Part model, mm, in its own coordinate system. Face numbers are marked on the shaded views. A direction names the side the tool comes from. Coordinates: 2 decimals unless noted, no trailing zeros. Order: outer loops, then holes, each group sorted by start corner. A loop starts at its lowest first (then second) coordinate and runs counter-clockwise, first axis right, second up.
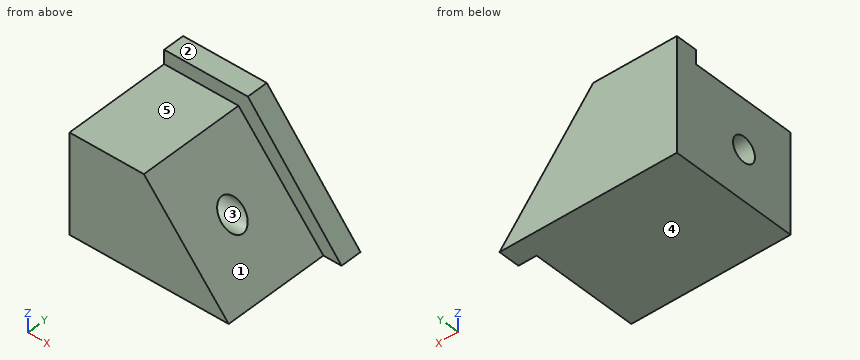
from build123d import *

# Parameters (mm, degrees)
F1_DEPTH = 76.2
F2_DEPTH = 12.7
F3_R     = 7.356687
F4_DEPTH = 104.797916


with BuildPart() as f1:
    # F0 (on Front) → F1 (new body)
    with BuildSketch(Plane.XZ):
        Polygon((0, 58.801956), (0, 0), (94.055586, 0), (43.929327, 58.801956), align=None)
    extrude(amount=F1_DEPTH)

    # F0 (on Front) → F2 (join)
    with BuildSketch(Plane.XZ):
        Polygon((0, 67.064524), (0, 58.801956), (43.929327, 58.801956), (94.055586, 0), (104.796916, 0), (49.437713, 67.064524), align=None)
    extrude(amount=F2_DEPTH)

    # F3 (on Right) → F4 (cut, through all)
    with BuildSketch(Plane.YZ):
        with Locations((-44.999432, 29.680481)):
            Circle(F3_R)
    extrude(amount=F4_DEPTH, mode=Mode.SUBTRACT)


solid = f1.part
Q1. Cut at C-C on x = 15.5. Write the cut outline in (y, z), and give its area (3 significant figures).
Results list:
outline: (-76.2, 0) - (0, 0) - (0, 67.06) - (-12.7, 67.06) - (-12.7, 58.8) - (-76.2, 58.8) - close; hole circle Ø14.71 at (-45, 29.68)
area: 4,420 mm2
Q2. Cut at D-D on z = 52. Write the cut outline in (x, y).
Results list:
outline: (0, -76.2) - (49.73, -76.2) - (49.73, -12.7) - (61.87, -12.7) - (61.87, 0) - (0, 0) - close
Q3. Pin check, flat tips, straight feed: pin 1 Ø1 at (x, y) = (87.5, -61.5) entering from +Z; pin 2 Ø8 at (y, z) = (-42.5, 47.5) entering from +X. Stop position of each tip, or through.
Results list:
pin 1: stops at z = 8.28
pin 2: stops at x = 56.97
Q4. Mould opens along Z. For the marked faces 3, 4 and 5 say: pulls with the +Z half, pulls with the -Z half, needs draft (parallel to the pull), parting line crosses it, or undercut.
Results list:
face 3: undercut
face 4: pulls with the -Z half
face 5: pulls with the +Z half
Q5. Which spindle directions (+Z, -Z, +X, -X, +Y, -Y) get a long thin tool onto all of the face, cutting with end or side? Do the marked faces 1 and 2. Say none if no direction does.
Results list:
face 1: +Z, +X, -Y
face 2: +Z, +X, -X, +Y, -Y
Q6. Wall check: line 1 along Z through (x, y) = (12, -45.5); line 2 along Z through (x, y) = (36, -63); line 3 along Y through (x, z) = (82, 22). Give the ranges that are in metal, low to high.
Results list:
line 1: z = 0 to 22.34, 37.02 to 58.8
line 2: z = 0 to 58.8
line 3: y = -12.7 to 0
Q7. Cut at A-A on z = 28. Write the cut outline in (x, y), and give its area (3 significant figures).
Results list:
outline: (0, -76.2) - (70.19, -76.2) - (70.19, -52.16) - (0, -52.16) - close; (0, -37.84) - (70.19, -37.84) - (70.19, -12.7) - (81.68, -12.7) - (81.68, 0) - (0, 0) - close
area: 4,490 mm2
Q8. Cut at B-B on y = -50. Write the cut outline in (x, z).
Results list:
outline: (0, 0) - (94.06, 0) - (73.35, 24.28) - (0, 24.28) - close; (0, 35.08) - (64.15, 35.08) - (43.93, 58.8) - (0, 58.8) - close
